Input: part model. Units: mm. Frame: model coordinates. A direction names the side the tool comes from. Give positions to 0.01 mm unless a question says otherwise; leave off trailing zeros. Write each loop counter-clockwise with the first axis right and the second up, starting at its lowest first coordinate (ties: lowest second). Pieces come first, ordered by that corner, then holes. Notation, with made-up numbers: (-40, -19.5) -> (17, -19.5) arc R16 cw to (17, 8.5) -> close; hole circle Ø9 at (21.5, 69.5). An arc over 180 degrees is marked (long way). Answer as a JSON object with one key per item and string values. Group by question number.
Autodesk Inventor part; units mm, degrees
ref_plane "YZ Plane" through (0, 0, 0) normal (1, 0, 0) x (0, 1, 0)
ref_plane "XZ Plane" through (0, 0, 0) normal (0, 1, 0) x (-1, 0, 0)
ref_plane "XY Plane" through (0, 0, 0) normal (0, 0, 1) x (1, 0, 0)
sketch "Sketch1" plane through (0, 0, 0) normal (0, 1, 0) x (-1, 0, 0)
  line L0 (-22.5, 37.5) -> (22.5, 37.5)
  line L1 (22.5, 37.5) -> (22.5, -37.5)
  line L2 (22.5, -37.5) -> (-22.5, -37.5)
  line L3 (-22.5, -37.5) -> (-22.5, 37.5)
  line L4 (22.5, 37.5) -> (-22.5, -37.5) construction
  line L5 (-20, 35) -> (20, 35)
  line L6 (20, 35) -> (20, -35)
  line L7 (20, -35) -> (-20, -35)
  line L8 (-20, -35) -> (-20, 35)
  line L9 (20, 35) -> (-20, -35) construction
  line L10 (20, 35) -> (17.5, 35)
  line L11 (17.5, 35) -> (17.5, 32.5)
  line L12 (17.5, 32.5) -> (20, 32.5)
  line L13 (20, 32.5) -> (20, 35)
  arc A0 (20, 32.5) -> (17.5, 35) centre (17.5, 32.5) ccw
  line L14 (22.5, 37.5) -> (19, 37.5)
  line L15 (19, 37.5) -> (19, 34)
  line L16 (19, 34) -> (22.5, 34)
  line L17 (22.5, 34) -> (22.5, 37.5)
  line L18 (20, -35) -> (17.5, -35)
  line L19 (17.5, -35) -> (17.5, -32.5)
  line L20 (17.5, -32.5) -> (20, -32.5)
  line L21 (20, -32.5) -> (20, -35)
  line L22 (-20, -35) -> (-17.5, -35)
  line L23 (-17.5, -35) -> (-17.5, -32.5)
  line L24 (-17.5, -32.5) -> (-20, -32.5)
  line L25 (-20, -32.5) -> (-20, -35)
  line L26 (-20, 35) -> (-17.5, 35)
  line L27 (-17.5, 35) -> (-17.5, 32.5)
  line L28 (-17.5, 32.5) -> (-20, 32.5)
  line L29 (-20, 32.5) -> (-20, 35)
  arc A1 (-17.5, 35) -> (-20, 32.5) centre (-17.5, 32.5) ccw
  arc A2 (-20, -32.5) -> (-17.5, -35) centre (-17.5, -32.5) ccw
  arc A3 (17.5, -35) -> (20, -32.5) centre (17.5, -32.5) ccw
  arc A4 (22.5, 34) -> (19, 37.5) centre (19, 34) ccw
  line L30 (22.5, -37.5) -> (19, -37.5)
  line L31 (19, -37.5) -> (19, -34)
  line L32 (19, -34) -> (22.5, -34)
  line L33 (22.5, -34) -> (22.5, -37.5)
  line L34 (-22.5, -37.5) -> (-19, -37.5)
  line L35 (-19, -37.5) -> (-19, -34)
  line L36 (-19, -34) -> (-22.5, -34)
  line L37 (-22.5, -34) -> (-22.5, -37.5)
  line L38 (-22.5, 37.5) -> (-19, 37.5)
  line L39 (-19, 37.5) -> (-19, 34)
  line L40 (-19, 34) -> (-22.5, 34)
  line L41 (-22.5, 34) -> (-22.5, 37.5)
  arc A5 (-19, 37.5) -> (-22.5, 34) centre (-19, 34) ccw
  arc A6 (-22.5, -34) -> (-19, -37.5) centre (-19, -34) ccw
  arc A7 (19, -37.5) -> (22.5, -34) centre (19, -34) ccw
  point P0 (0, 0)
  point P1 (-19.5, -34)
  point P2 (-20, -34)
  dimension "d0" = 45
  dimension "d1" = 75
  dimension "d2" = 40
  dimension "d3" = 70
  dimension "d8" = 2.5
  dimension "d9" = 2.5
extrude "Extrusion3" add sketch "Sketch1" along normal blind 2.5 contours L0 L15 L5 L39 | L39 L5 L8 L40 A5 | L40 L8 L36 L3 | A4 L16 L6 L5 L15 | L39 A1 L40 L8 L5 | L5 A1 L39 | L36 L8 L7 L35 A6 | L40 A1 L8 | L15 A0 L5 | L5 L6 L16 A0 L15 | L1 L32 L6 L16 | L5 L11 L12 L6 L20 L19 L7 L23 L24 L8 L28 L27 | L27 L28 A1 L40 L39 | L39 L40 A1 | L36 A2 L35 L7 L8 | L35 L7 L31 L2 | A0 L15 L16 L12 L11 | A0 L16 L15 | A7 L31 L7 L6 L32 | L6 A0 L16 | L24 L23 A2 L35 L36 | L36 L35 A2 | L35 A2 L7 | L32 A3 L6 | L6 L7 L31 A3 L32 | L7 A3 L31 | A3 L32 L31 L19 L20 | A3 L31 L32
extrude "Extrusion4" add sketch "Sketch1" along normal blind 37.5 contours L0 L15 L5 L39 | L39 L5 L8 L40 A5 | L40 L8 L36 L3 | A4 L16 L6 L5 L15 | L39 A1 L40 L8 L5 | L5 A1 L39 | L36 L8 L7 L35 A6 | L40 A1 L8 | L15 A0 L5 | L5 L6 L16 A0 L15 | L1 L32 L6 L16 | L36 A2 L35 L7 L8 | L8 A2 L36 | L35 L7 L31 L2 | A7 L31 L7 L6 L32 | L6 A0 L16 | L35 A2 L7 | L32 A3 L6 | L6 L7 L31 A3 L32 | L7 A3 L31
fillet "Fillet1" radius 3 8 edges at (-21.4749, 0, 36.4749) (0, 0, 37.5) (21.4749, 0, 36.4749) (22.5, 0, 0) (21.4749, 0, -36.4749) (0, 0, -37.5) (-21.4749, 0, -36.4749) (-22.5, 0, 0)
sketch "Sketch2" plane through (0, 2.5, 0) normal (0, 1, 0) x (1, 0, 0)
  arc A0 (20, 32.5) -> (17.5, 35) centre (17.5, 32.5) ccw
  line L0 (17.5, 35) -> (17.5, 33.5)
  line L1 (20, -32.5) -> (20, 32.5)
  line L2 (20, 32.5) -> (18.5, 32.5)
  line L3 (18.5, 32.5) -> (17.5, 33.5)
  line L4 (18, 33) -> (16.0555, 31.0555)
  circle A1 centre (16.0555, 31.0555) radius 2.75
  line L5 (-20, 32.5) -> (-20, -32.5)
  line L6 (-20, -32.5) -> (-18.5, -32.5)
  line L7 (-17.5, -35) -> (17.5, -35)
  line L8 (-17.5, -35) -> (-17.5, -33.5)
  line L9 (-17.5, -33.5) -> (-18.5, -32.5)
  line L10 (-18, -33) -> (-16.0555, -31.0555)
  line L11 (-18, -33) -> (-15.25, -33) construction
  circle A2 centre (-16.0555, -31.0555) radius 2.75
  arc A3 (17.5812, 28.7675) -> (18.8055, 31.0555) centre (16.0555, 31.0555) ccw construction
  arc A4 (17.8504, 28.3639) -> (19.2906, 31.0555) centre (16.0555, 31.0555) ccw
  arc A5 (17.3121, 29.1712) -> (18.3203, 31.0555) centre (16.0555, 31.0555) ccw
  arc A6 (17.3121, 29.1712) -> (17.8504, 28.3639) centre (17.5812, 28.7675) ccw
  arc A7 (19.2906, 31.0555) -> (18.3203, 31.0555) centre (18.8055, 31.0555) ccw
  arc A8 (14.2605, 33.747) -> (12.8203, 31.0555) centre (16.0555, 31.0555) ccw
  arc A9 (12.8203, 31.0555) -> (13.7906, 31.0555) centre (13.3055, 31.0555) ccw
  arc A10 (14.7989, 32.9398) -> (14.2605, 33.747) centre (14.5297, 33.3434) ccw
  arc A11 (14.7989, 32.9398) -> (13.7906, 31.0555) centre (16.0555, 31.0555) ccw
  arc A12 (-14.2605, -33.747) -> (-12.8203, -31.0555) centre (-16.0555, -31.0555) ccw
  arc A13 (-14.7989, -32.9398) -> (-13.7906, -31.0555) centre (-16.0555, -31.0555) ccw
  arc A14 (-14.7989, -32.9398) -> (-14.2605, -33.747) centre (-14.5297, -33.3434) ccw
  arc A15 (-12.8203, -31.0555) -> (-13.7906, -31.0555) centre (-13.3055, -31.0555) ccw
  arc A16 (-17.8504, -28.3639) -> (-19.2906, -31.0555) centre (-16.0555, -31.0555) ccw
  arc A17 (-19.2906, -31.0555) -> (-18.3203, -31.0555) centre (-18.8055, -31.0555) ccw
  arc A18 (-17.3121, -29.1712) -> (-17.8504, -28.3639) centre (-17.5812, -28.7675) ccw
  arc A19 (-17.3121, -29.1712) -> (-18.3203, -31.0555) centre (-16.0555, -31.0555) ccw
  line L12 (-19.2843, -34.2843) -> (-16.7157, -31.7157) construction
  line L13 (-18.86, -34.7085) -> (-16.2915, -32.14)
  line L14 (-17.14, -31.2915) -> (-19.7085, -33.86)
  arc A20 (-19.7085, -33.86) -> (-18.86, -34.7085) centre (-19.2843, -34.2843) ccw
  arc A21 (-16.2915, -32.14) -> (-17.14, -31.2915) centre (-16.7157, -31.7157) ccw
  line L15 (16.5205, 31.5205) -> (19.4795, 34.4795) construction
  line L16 (16.9448, 31.0962) -> (19.9038, 34.0552)
  line L17 (19.0552, 34.9038) -> (16.0962, 31.9448)
  arc A22 (16.0962, 31.9448) -> (16.9448, 31.0962) centre (16.5205, 31.5205) ccw
  arc A23 (19.9038, 34.0552) -> (19.0552, 34.9038) centre (19.4795, 34.4795) ccw
  point P0 (0, 0)
  point P1 (18.3774, 32.5289)
  point P2 (17.5289, 33.3774)
  point P3 (14.9555, 33.5759)
  point P4 (13.3482, 30.5722)
  point P5 (17.1554, 28.535)
  point P6 (18.7627, 31.5387)
  point P7 (-18.3774, -32.5289)
  point P8 (-17.5289, -33.3774)
  point P9 (-14.9555, -33.5759)
  point P10 (-13.3482, -30.5722)
  point P11 (-17.1554, -28.535)
  point P12 (-18.7627, -31.5387)
  point P13 (18.7918, 34.6404)
  point P14 (19.6404, 33.7918)
  dimension "d32" = 5.5
  dimension "d29" = 1.5
  dimension "d30" = 1.5
  dimension "d31" = 2.75
  dimension "d33" = 1.5
  dimension "d34" = 1.5
  dimension "d35" = 2.75
  dimension "d36" = 45
  dimension "d37" = 5.5
  dimension "d40" = 360
  dimension "d44" = 1.2
  dimension "d45" = 1.2
extrude "Extrusion5" add sketch "Sketch2" along normal blind 35 contours A0 L17 A23 L16 | A1 L16 A22 L4 | L4 A22 L17 A1 | A1 A7 A5 A6 A9 A11 A10 L17 A22 L16 | A1 A6 A5 A7 | A10 A11 A9 A1 | A2 L14 A21 L10 | L10 A21 L13 A2 | L13 A21 L14 A2 A17 A19 A18 A15 A13 A14 | A14 A13 A15 A2 | A2 A18 A19 A17
extrude "Extrusion6" add sketch "Sketch2" along normal blind 10 contours A7 A4 A6 A1 | A1 A9 A8 A10 | A2 L14 A21 L10 | L10 A21 L13 A2 | L13 A21 L14 A2 A17 A19 A18 A15 A13 A14 | A14 A13 A15 A2 | A2 A15 A12 A14 | A17 A16 A18 A2 | A2 A18 A19 A17
sketch "Sketch3" plane through (0, 37.5, 0) normal (0, 1, 0) x (1, 0, 0)
  arc A0 (-13.3055, -31.0555) -> (-13.3055, -31.0555) centre (-16.0555, -31.0555) ccw
  circle A1 centre (-16.0555, -31.0555) radius 1.5
  circle A2 centre (-16.0555, -31.0555) radius 1.25
  circle A3 centre (16.0488, 31.0622) radius 1.5
  circle A4 centre (16.0488, 31.0622) radius 1.25
  point P0 (0, 0)
  dimension "d50" = 3
  dimension "d51" = 2.5
  dimension "d52" = 3
  dimension "d53" = 2.5
extrude "Extrusion7" cut sketch "Sketch3" against normal blind 0.5 contours A1 | A3
extrude "Extrusion8" cut sketch "Sketch3" against normal blind 20 contours A2 | A4
extrude "Extrusion9" add sketch "Sketch2" along normal blind 32 contours L16 L3 L17 A0 | L16 A1 L3 | L3 A1 L17 | L13 A20 L14 L9 | L9 A2 L13 | L9 L14 A2
properties part number "proper shit spodnji"
1. Section B-B (z = -4). Return the cut outline in (x, y), plus the area to 3 significant figures.
2. Section A-A (y = 16). Return the cut outline in (x, z), plus the area to 3 significant figures.
3. Section C-C (x = -3). Return the cut outline in (y, z), plus the area to 3 significant figures.
4. Line query: line 1 (X direction, y = 21, z = 15); line 2 (X direction, y = 36, z = -29); line 3 (Z direction, x = 5, y = 8). Output: solid intervals per line, ascending.
5. Section D-D (y = 27.5). Return the cut outline in (x, z), plus the area to 3 significant figures.
6. Mould query, pull axis X, two halves, no side actions, for faces 1 (the face through (-21.45, 20.01, 36.5)), 2 (the face through (22.5, 20, 0)), 3 (the face through (13.4, 12.5, -32.3)), 4 (the face through (17.24, 37.5, -29.87)). Classes: pulls with the +X half, pulls with the -X half, needs draft (parallel to the pull), parting line crosses it, or undercut.
7. Contact query for a flat-ended pin moving along its axis: pin 1 Ø1.2 at (x, z) = (-16, 30.5) entering from +Y. Output: stop coordinate, or through.
8. Reachability of faces 5 (the face through (-22.5, 20, 0)), 6 (the face through (0, 20, 35)) from +Z, -Z, +X, -X, +Y, -Y: full face, straight path, thin tool, end or side. Return the list, or none.
Working result:
{
 "1": {"outline": "(-22.5, 3) arc R3 ccw to (-19.5, 0) -> (19.5, 0) arc R3 ccw to (22.5, 3) -> (22.5, 37.5) -> (20, 37.5) -> (20, 2.5) -> (-20, 2.5) -> (-20, 37.5) -> (-22.5, 37.5) -> close", "area": "284 mm^2"},
 "2": {"outline": "(-22.5, -34) arc R3.5 ccw to (-19, -37.5) -> (19, -37.5) arc R3.5 ccw to (22.5, -34) -> (22.5, 34) arc R3.5 ccw to (19, 37.5) -> (-19, 37.5) arc R3.5 ccw to (-22.5, 34) -> close; hole (-20, -32.5) arc R2.5 ccw to (-17.5, -35) -> (17.5, -35) arc R2.5 ccw to (18.79, -34.64) -> (17.53, -33.38) arc R2.75 cw (long way) to (18.38, -32.53) -> (19.64, -33.79) arc R2.5 ccw to (20, -32.5) -> (20, 32.5) arc R2.5 ccw to (17.5, 35) -> (-17.5, 35) arc R2.5 ccw to (-18.79, 34.64) -> (-17.53, 33.38) arc R2.75 cw (long way) to (-18.38, 32.53) -> (-19.64, 33.79) arc R2.5 ccw to (-20, 32.5) -> close", "area": "622 mm^2"},
 "3": {"outline": "(0, -34.5) arc R3 ccw to (3, -37.5) -> (37.5, -37.5) -> (37.5, -35) -> (2.5, -35) -> (2.5, 35) -> (37.5, 35) -> (37.5, 37.5) -> (3, 37.5) arc R3 ccw to (0, 34.5) -> close", "area": "359 mm^2"},
 "4": {"line 1": "x = -22.5 to -20, 20 to 22.5", "line 2": "x = -22.5 to -20, 14.23 to 17.88, 20 to 22.5", "line 3": "z = -37.5 to -35, 35 to 37.5"},
 "5": {"outline": "(-22.5, -34) arc R3.5 ccw to (-19, -37.5) -> (19, -37.5) arc R3.5 ccw to (22.5, -34) -> (22.5, 34) arc R3.5 ccw to (19, 37.5) -> (-19, 37.5) arc R3.5 ccw to (-22.5, 34) -> close; hole (-20, -32.5) arc R2.5 ccw to (-17.5, -35) -> (17.5, -35) arc R2.5 ccw to (18.79, -34.64) -> (17.53, -33.38) arc R2.75 cw (long way) to (18.38, -32.53) -> (19.64, -33.79) arc R2.5 ccw to (20, -32.5) -> (20, 32.5) arc R2.5 ccw to (17.5, 35) -> (-17.5, 35) arc R2.5 ccw to (-18.79, 34.64) -> (-17.53, 33.38) arc R2.75 cw (long way) to (-18.38, 32.53) -> (-19.64, 33.79) arc R2.5 ccw to (-20, 32.5) -> close; hole circle Ø2.5 at (-16.06, 31.06); hole circle Ø2.5 at (16.05, -31.06)", "area": "612 mm^2"},
 "6": {"face 1": "pulls with the -X half", "face 2": "pulls with the +X half", "face 3": "undercut", "face 4": "needs draft"},
 "7": {"pin 1": "stops at y = 17.5"},
 "8": {"face 5": "+Z, -Z, -X, +Y, -Y", "face 6": "+Y"}
}
